Source: three-view drawing plus pictorial views. Frame: mm from the lowest corner of the part. A direction names the side the tool comes from. Give positions to 0.01 mm unless a question says otherwise; leave off trailing zeros. Order: outer loops, then holes, each group sorted by start corner. A loop starts at its lowest first (then second) coordinate and runs counter-clockwise, first axis right, second up. Notation, with made-up numbers: (-35, -31) -> (2, -31) arc R16 cw to (2, -16) -> close; hole circle Ø11 at (0, 68). An arc over 180 degrees is marked (long way). Write item = value, one per line.
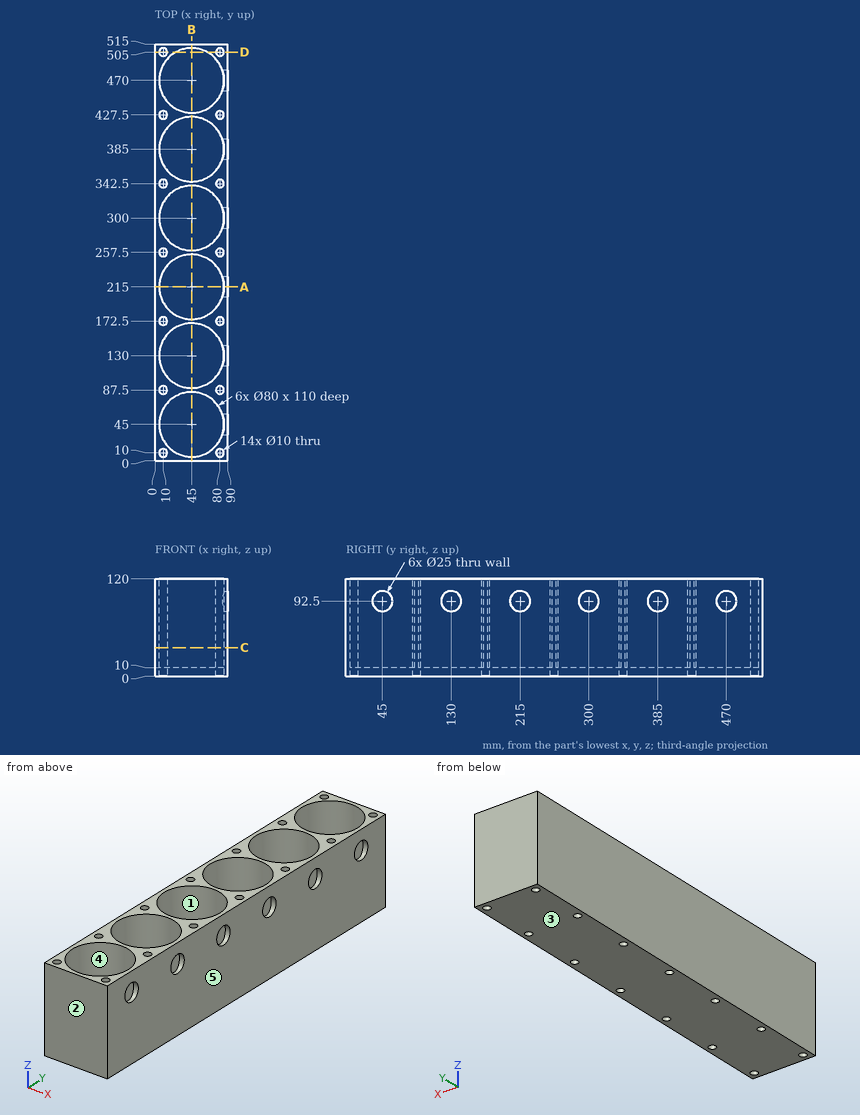
1) First-contact query: P1, Ø9, axis at x = 80, y = 427.5, coming from the +Z side; P2, Ø24, axis at x = 58, y = 112.5, coming from the +Z side. Flat tips, straight axial feed; report the tip coordinate or a pass-through.
Check sheet entries:
P1 = through
P2 = 10
2) Line query: line 1 (X direction, y = 87.5, z = 64); line 2 (Z direction, x = 85.5, y = 470); line 3 (X direction, y = 131, z = 107). Output: solid intervals per line, ascending. Write a range as from..to.
Check sheet entries:
line_1 = 0..5, 15..75, 85..90
line_2 = 0..80, 105..120
line_3 = 0..5.01, 84.99..90
3) Section query B-B (x = 45). Output: boundary loops of the cut face in (y, z), plus the area to 3 significant figures.
Check sheet entries:
outline = (0, 0) -> (515, 0) -> (515, 120) -> (510, 120) -> (510, 10) -> (430, 10) -> (430, 120) -> (425, 120) -> (425, 10) -> (345, 10) -> (345, 120) -> (340, 120) -> (340, 10) -> (260, 10) -> (260, 120) -> (255, 120) -> (255, 10) -> (175, 10) -> (175, 120) -> (170, 120) -> (170, 10) -> (90, 10) -> (90, 120) -> (85, 120) -> (85, 10) -> (5, 10) -> (5, 120) -> (0, 120) -> close
area = 9,000 mm²
4) Section query D-D (y = 505). Output: boundary loops of the cut face in (x, z).
Check sheet entries:
outline = (0, 0) -> (5, 0) -> (5, 120) -> (0, 120) -> close; (15, 0) -> (75, 0) -> (75, 120) -> (64.36, 120) -> (64.36, 10) -> (25.64, 10) -> (25.64, 120) -> (15, 120) -> close; (85, 0) -> (90, 0) -> (90, 120) -> (85, 120) -> close
5) Mould query, pull axis Y, two halves, no side actions, for the marked faces 1, 2 and 3. Classes: +Y half, -Y half, draft (parallel to the pull), parting line (faces both ways), or undercut.
Check sheet entries:
face_1 = undercut
face_2 = -Y half
face_3 = draft
6) Reachability of the marked faces 4 and 5 from +Z, -Z, +X, -X, +Y, -Y: full face, straight path, thin tool, end or side. Return the list, or none.
Check sheet entries:
face_4 = +Z
face_5 = +Z, -Z, +X, +Y, -Y
7) Section query C-C (z = 35). Count the separate pieces of the cut face and the enclosed holes in it, plus the area to 3 significant figures.
Check sheet entries:
separate_pieces = 1
enclosed_holes = 20
area = 15,100 mm²
8) Section query A-A (y = 215). Output: boundary loops of the cut face in (x, z).
Check sheet entries:
outline = (0, 0) -> (90, 0) -> (90, 80) -> (85, 80) -> (85, 10) -> (5, 10) -> (5, 120) -> (0, 120) -> close; (85, 105) -> (90, 105) -> (90, 120) -> (85, 120) -> close
